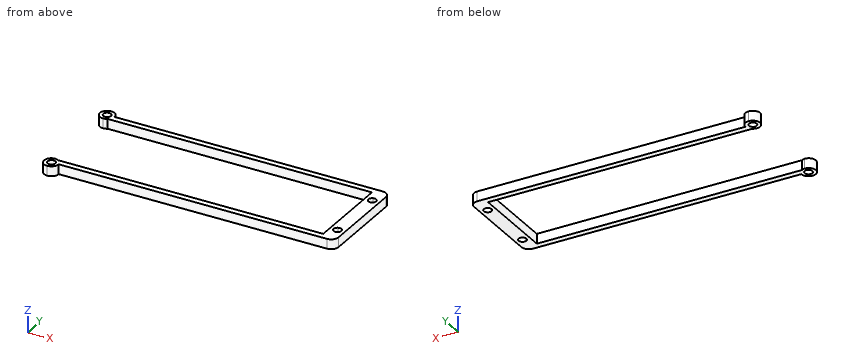
```python
from build123d import *

# Parameters (mm, degrees)
SKETCH1_R           = 1.6
BOSS_EXTRUDE1_DEPTH = 4
SKETCH2_R           = 1.6
BOSS_EXTRUDE2_DEPTH = 4
SKETCH3_R           = 1.6
CUT_EXTRUDE1_DEPTH  = 4
SKETCH4_W           = 1
SKETCH4_H           = 46
BOSS_EXTRUDE4_DEPTH = 4
SKETCH6_R           = 1.6
SKETCH6_W           = 1
SKETCH6_H           = 34
CUT_EXTRUDE2_DEPTH  = 4
CUT_EXTRUDE4_DEPTH  = 4
FILLET2_R           = 3
CUT_EXTRUDE5_DEPTH  = 10
FILLET3_R           = 3


with BuildPart() as part:
    # Sketch1 → Boss-Extrude1 (new body)
    with BuildSketch(Plane.XY):
        with BuildLine():
            Line((0, 34), (106, 34))
            Line((106, 34), (106, 0))
            Line((106, 0), (0, 0))
            Line((0, 0), (-3, 0))
            ThreePointArc((-3, 0), (-6, -3), (-3, -6))
            Line((-3, -6), (112, -6))
            Line((112, -6), (112, 0))
            Line((112, 0), (112, 40))
            Line((112, 40), (-3, 40))
            ThreePointArc((-3, 40), (-6, 37), (-3, 34))
            Line((-3, 34), (0, 34))
        make_face()
        with Locations((-3, 37)):
            Circle(SKETCH1_R, mode=Mode.SUBTRACT)
        with Locations((-3, -3)):
            Circle(SKETCH1_R, mode=Mode.SUBTRACT)
        with Locations((109, 29.25)):
            Circle(SKETCH1_R, mode=Mode.SUBTRACT)
        with Locations((109, 4.75)):
            Circle(SKETCH1_R, mode=Mode.SUBTRACT)
    extrude(amount=BOSS_EXTRUDE1_DEPTH)

    # Sketch2 → Boss-Extrude2 (add)
    with BuildSketch(Plane.XY.offset(4)):
        with Locations((109, 4.75)):
            Circle(SKETCH2_R)
        with Locations((109, 29.25)):
            Circle(SKETCH2_R)
    extrude(amount=-BOSS_EXTRUDE2_DEPTH)

    # Sketch3 → Cut-Extrude1 (cut)
    with BuildSketch(Plane.XY.offset(4)):
        with Locations((109, 29.5)):
            Circle(SKETCH3_R)
        with Locations((109, 4.5)):
            Circle(SKETCH3_R)
    extrude(amount=-CUT_EXTRUDE1_DEPTH, mode=Mode.SUBTRACT)

    # Sketch4 → Boss-Extrude4 (add)
    with BuildSketch(Plane.XY.offset(4)):
        with Locations((112.5, 17)):
            Rectangle(SKETCH4_W, SKETCH4_H)
        with BuildLine():
            ThreePointArc((109.5, 27.980131585), (108.4, 29.5), (109.5, 31.019868415))
            ThreePointArc((109.5, 31.019868415), (107.4, 29.5), (109.5, 27.980131585))
        make_face()
        with BuildLine():
            ThreePointArc((109.566346567, 3.003587101), (108.401525498, 4.473847256), (109.433653433, 6.040111912))
            ThreePointArc((109.433653433, 6.040111912), (107.401525498, 4.430148243), (109.566346567, 3.003587101))
        make_face()
    extrude(amount=-BOSS_EXTRUDE4_DEPTH)

    # Sketch6 → Cut-Extrude2 (cut)
    with BuildSketch(Plane.XY.offset(4)):
        with Locations((110, 4.543699012)):
            Circle(SKETCH6_R)
        with Locations((110, 29.5)):
            Circle(SKETCH6_R)
        with Locations((106.5, 17)):
            Rectangle(SKETCH6_W, SKETCH6_H)
    extrude(amount=-CUT_EXTRUDE2_DEPTH, mode=Mode.SUBTRACT)

    # Sketch7 → Cut-Extrude4 (cut)
    with BuildSketch(Plane.XY.offset(4)):
        with BuildLine():
            Line((52, 0), (-3, 0))
            ThreePointArc((-3, 0), (-2.373132959, -0.184325643), (-1.801042119, -0.5))
            Line((-1.801042119, -0.5), (52, -0.5))
            Line((52, -0.5), (107, -0.5))
            Line((107, -0.5), (107, 0))
            Line((107, 0), (52, 0))
        make_face()
        with BuildLine():
            Line((52, 34.5), (-1.341687605, 34.5))
            ThreePointArc((-1.341687605, 34.5), (-2.133974596, 34.127718677), (-3, 34))
            Line((-3, 34), (52, 34))
            Line((52, 34), (107, 34))
            Line((107, 34), (107, 34.5))
            Line((107, 34.5), (52, 34.5))
        make_face()
    extrude(amount=-CUT_EXTRUDE4_DEPTH, mode=Mode.SUBTRACT)

    # Fillet2
    fillet2_edges = [part.edges().sort_by_distance(p)[0] for p in [
        (113, -6, 2),
        (113, 40, 2),
    ]]
    fillet(fillet2_edges, radius=FILLET2_R)

    # Sketch8 → Cut-Extrude5 (cut)
    with BuildSketch(Plane.XY.offset(4)):
        with BuildLine():
            Line((0, 37), (113, 37))
            Line((113, 37), (119.400968333, 46.55128084))
            Line((119.400968333, 46.55128084), (-5.470878247, 48.639937772))
            Line((-5.470878247, 48.639937772), (-3, 40))
            ThreePointArc((-3, 40), (-0.878679656, 39.121320344), (0, 37))
        make_face()
        with BuildLine():
            Line((0, -3), (113, -3))
            Line((113, -3), (122.38476395, -22.523587699))
            Line((122.38476395, -22.523587699), (1.093472111, -19.390602301))
            Line((1.093472111, -19.390602301), (-3, -6))
            ThreePointArc((-3, -6), (-0.878679656, -5.121320344), (0, -3))
        make_face()
    extrude(amount=-CUT_EXTRUDE5_DEPTH, mode=Mode.SUBTRACT)

    # Fillet3
    fillet3_edges = [part.edges().sort_by_distance(p)[0] for p in [
        (113, -3, 2),
        (113, 37, 2),
    ]]
    fillet(fillet3_edges, radius=FILLET3_R)


solid = part.part
```
Can you work these out from the model? Positions are in its coordinate system, mm. Give positions to 0.01 mm unless a question says otherwise; leave off trailing zeros. Loops run counter-clockwise (first coordinate to the right, second up) from the corner with the lowest first, then second, coordinate; pieces in that order, holes last. Notation, with made-up numbers: M 35,-29 L 77,-29 A16 cw 77,-8 Z; hole C 71,59 d10. An arc over 180 degrees is marked long. Use one line per item in the form item = value. Start each with the question number.
(1) Please list where these lines run through material, in increasing order: line 1 (Y direction, x = 110, z = 1.25); line 2 (Y direction, x = -3, z = 1.6); line 3 (X direction, y = 29.5, z = 3.4).
(2) I want a section at A-A, the plane z = 3.15. Write out the boundary of the cut face in (x, y).
(3) I want a section at C-C, the plane x = 49.5. Write out the boundary of the cut face in (y, z), and give its area (3 significant figures).
(4) I'm going to push flat-ended pins straight in: P1, Ø2, axis at x = 27, z = 1.5, coming from the +Y side; P2, Ø1.5, axis at x = 97.5, z = 1.5, coming from the -Y side; P3, Ø5, axis at x = -3, y = 37, coming from the +Z side; P4, Ø3, axis at x = 110, y = 29.5, coming from the +Z side. Where does each tip first touch, or does it pass through?
(5) I want a section at B-B, the plane y = 29.5. Write out the boundary of the cut face in (x, z), and give its area (3 significant figures).
Worked out:
q1.line_1 = -3 to 2.94, 6.14 to 27.9, 31.1 to 37
q1.line_2 = -6 to -4.6, -1.4 to 0, 34 to 35.4, 38.6 to 40
q1.line_3 = 107 to 108.4, 111.6 to 113
q2.outline = M -3,0 A3 ccw long 0,-3 L 110,-3 A3 ccw 113,0 L 113,34 A3 ccw 110,37 L 0,37 A3 ccw long -1.34,34.5 L 107,34.5 L 107,-0.5 L -1.8,-0.5 A3 ccw Z; hole C -3,-3 d3.2; hole C -3,37 d3.2; hole C 110,4.54 d3.2; hole C 110,29.5 d3.2
q3.outline = M -3,0 L -0.5,0 L -0.5,4 L -3,4 Z; M 34.5,0 L 37,0 L 37,4 L 34.5,4 Z
q3.area = 20.0 mm²
q4.P1 = 37
q4.P2 = -3
q4.P3 = 4
q4.P4 = through
q5.outline = M 107,0 L 108.4,0 L 108.4,4 L 107,4 Z; M 111.6,0 L 113,0 L 113,4 L 111.6,4 Z
q5.area = 11.2 mm²
